Check sheet for the modelled part. Datum: model origin and axes. Units: mm. A direction names the side the tool comes from. Give positions to 0.01 mm unless a question says otherwise; leave off trailing zeros. Write each loop counter-clockwise with the first axis right and the second up, starting at its lowest first coordinate (ties: lowest second). Pieces come first, ordered by that corner, then holes. Notation, with made-up numbers: (30, 8.5) -> (73, 8.5) arc R24 ccw to (73, 20.5) -> close; hole circle Ø11 at (-1.75, -13). An arc over 180 degrees is marked (long way). Return JSON: item names as keys, results as strings.
from build123d import *

# Parameters (mm, degrees)
SKETCH1_W           = 30.2
SKETCH1_H           = 28.8
BOSS_EXTRUDE1_DEPTH = 6.9
SKETCH2_R           = 2.1
BOSS_EXTRUDE2_DEPTH = 5
SKETCH3_W           = 2
SKETCH3_H           = 8
BOSS_EXTRUDE3_DEPTH = 6.9
SKETCH4_W           = 2
SKETCH4_H           = 8
BOSS_EXTRUDE4_DEPTH = 6.6


with BuildPart() as part:
    # Sketch1 → Boss-Extrude1 (new body, symmetric)
    with BuildSketch(Plane(origin=(0, 0, 0), x_dir=(1, 0, 0), z_dir=(0, 1, 0))):
        with Locations((15.1, 14.4)):
            Rectangle(SKETCH1_W, SKETCH1_H)
    extrude(amount=BOSS_EXTRUDE1_DEPTH, both=True)

    # Sketch2 → Boss-Extrude2 (add)
    with BuildSketch(Plane(origin=(30.2, 0, 0), x_dir=(0, 0, -1), z_dir=(1, 0, 0))):
        with Locations((5, 0)):
            Circle(SKETCH2_R)
    extrude(amount=BOSS_EXTRUDE2_DEPTH)

    # Sketch3 → Boss-Extrude3 (add)
    with BuildSketch(Plane.XY):
        with Locations((28.2, 0)):
            Rectangle(SKETCH3_W, SKETCH3_H)
    extrude(amount=BOSS_EXTRUDE3_DEPTH)

    # Sketch4 → Boss-Extrude4 (add)
    with BuildSketch(Plane(origin=(0, 0, -28.8), x_dir=(-1, 0, 0), z_dir=(0, 0, -1))):
        with Locations((-28.2, 0)):
            Rectangle(SKETCH4_W, SKETCH4_H)
    extrude(amount=BOSS_EXTRUDE4_DEPTH)


solid = part.part
(1) Cross-section at C-C on x = 15. Enter the section's corners in (y, z).
Reply:
{"outline": "(-6.9, -28.8) -> (6.9, -28.8) -> (6.9, 0) -> (-6.9, 0) -> close"}
(2) Cross-section at D-D on y = 3. Enter the section's corners in (x, z), then the cut area to 3 significant figures.
Reply:
{"outline": "(0, -28.8) -> (27.2, -28.8) -> (27.2, -35.4) -> (29.2, -35.4) -> (29.2, -28.8) -> (30.2, -28.8) -> (30.2, 0) -> (29.2, 0) -> (29.2, 6.9) -> (27.2, 6.9) -> (27.2, 0) -> (0, 0) -> close", "area": "897 mm^2"}
(3) Depth check by flat-ended pin: pin 1 Ø0.6 at (x, z) = (28.5, 5) entering from -Y; pin 2 Ø5.5 at (y, z) = (-0.5, -33) entering from +X; pin 3 Ø8 at (x, y) = (9.5, -2.5) entering from +Z. Enter the tip coordinate at first touch or a pass-through.
Reply:
{"pin 1": "y = -4", "pin 2": "x = 29.2", "pin 3": "z = 0"}
(4) Set-up check for faces 1 (the flat face through (28, 4, -32)), 2 (the flat face through (28, -4, 3)), 3 (the flat face through (27.2, 0, -32)), 4 (the flat face through (27.2, 0, 3)), 5 (the cylindrical face through (32.665, 0.631, -7.003)): record each of +Z, -Z, +X, -X, +Y, -Y from which the full face is reachable in a straight line by a thin tool's end or side.
Reply:
{"face 1": "-Z, +X, -X, +Y", "face 2": "+Z, +X, -X, -Y", "face 3": "-Z, -X, +Y, -Y", "face 4": "+Z, -X, +Y, -Y", "face 5": "+X"}
(5) Cross-section at A-A on y = 0. Enter the section's corners in (x, z).
Reply:
{"outline": "(0, -28.8) -> (27.2, -28.8) -> (27.2, -35.4) -> (29.2, -35.4) -> (29.2, -28.8) -> (30.2, -28.8) -> (30.2, -7.1) -> (35.2, -7.1) -> (35.2, -2.9) -> (30.2, -2.9) -> (30.2, 0) -> (29.2, 0) -> (29.2, 6.9) -> (27.2, 6.9) -> (27.2, 0) -> (0, 0) -> close"}
(6) Thickness scan on L1, parallel to X at y = 2.5, z = -13; L2, parallel to Z at x = 8.5, y = 3.5; L3, parallel to Z at x = 34, y = -1.25. Record the ranges inside material, lowest first.
Reply:
{"L1": "0 to 30.2", "L2": "-28.8 to 0", "L3": "-6.69 to -3.31"}
(7) Cross-section at B-B on z = -5. Enter the section's corners in (x, y).
Reply:
{"outline": "(0, -6.9) -> (30.2, -6.9) -> (30.2, -2.1) -> (35.2, -2.1) -> (35.2, 2.1) -> (30.2, 2.1) -> (30.2, 6.9) -> (0, 6.9) -> close"}
